Verification items for the finished model (mm, model axes). Face numbers are marked on the shaded views. Give positions to 0.01 mm unless a question says otherwise; leave off trailing zeros. Loops run counter-clockwise (first coordinate to the right, second up) from the corner with the lowest first, then second, coordinate; pieces in that order, holes last. Notation, with made-up numbers: M -7,34.25 L -3,34.25 A6 cw -3,39.25 Z; hole C -21,-4.5 d10. An arc over 180 degrees is marked long. Use a Markdown table: item, result.
from build123d import *

# Parameters (mm, degrees)
SKETCH1_W             = 34.925
SKETCH1_H             = 50.8
BOSS_EXTRUDE1_DEPTH   = 1.5875
F_4_CLEARANCE_HOLE1_D = 3.2639
SKETCH6_W             = 15.875
SKETCH6_H             = 5.588
BOSS_EXTRUDE2_DEPTH   = 1.5875
CUT_EXTRUDE1_DEPTH    = 36.604988506
CUT_EXTRUDE2_DEPTH    = 36.604988506
SKETCH9_W             = 9.573595876
SKETCH9_H             = 10.540114366
CUT_EXTRUDE3_DEPTH    = 36.604988506
FILLET1_R             = 1.016


with BuildPart() as part:
    # Sketch1 → Boss-Extrude1 (new body)
    with BuildSketch(Plane(origin=(0, 0, 0), x_dir=(1, 0, 0), z_dir=(0, 1, 0))):
        Rectangle(SKETCH1_W, SKETCH1_H)
    extrude(amount=BOSS_EXTRUDE1_DEPTH)

    # #4 Clearance Hole1 (through all)
    with Locations(Plane(origin=(0, 1.5875, 0), x_dir=(1, 0, 0), z_dir=(0, 1, 0))):
        with Locations((-14.2875, 22.225), (14.2875, 22.225), (14.2875, -22.225), (-14.2875, -22.225)):
            Hole(F_4_CLEARANCE_HOLE1_D / 2)

    # Sketch6 → Boss-Extrude2 (add)
    with BuildSketch(Plane(origin=(0, 1.5875, 0), x_dir=(1, 0, 0), z_dir=(0, 1, 0))):
        with Locations((0, -28.194)):
            Rectangle(SKETCH6_W, SKETCH6_H)
    extrude(amount=-BOSS_EXTRUDE2_DEPTH)

    # Sketch7 → Cut-Extrude1 (cut, through all)
    with BuildSketch(Plane(origin=(0, 1.5875, 0), x_dir=(1, 0, 0), z_dir=(0, 1, 0))):
        with BuildLine():
            Line((-15.875, 13.8303), (-20.9423, 13.8303))
            Line((-20.9423, 13.8303), (-20.9423, 8.763))
            Line((-20.9423, 8.763), (-20.9423, 3.6957))
            Line((-20.9423, 3.6957), (-15.875, 3.6957))
            ThreePointArc((-15.875, 3.6957), (-10.8077, 8.763), (-15.875, 13.8303))
        make_face()
        with BuildLine():
            Line((12.7, 13.8303), (17.7673, 13.8303))
            Line((17.7673, 13.8303), (17.7673, 8.763))
            Line((17.7673, 8.763), (17.7673, 3.6957))
            Line((17.7673, 3.6957), (12.7, 3.6957))
            ThreePointArc((12.7, 3.6957), (7.6327, 8.763), (12.7, 13.8303))
        make_face()
    extrude(amount=-CUT_EXTRUDE1_DEPTH, mode=Mode.SUBTRACT)

    # Sketch8 → Cut-Extrude2 (cut, through all)
    with BuildSketch(Plane(origin=(0, 1.5875, 0), x_dir=(1, 0, 0), z_dir=(0, 1, 0))):
        with BuildLine():
            Line((6.604, -14.342881029), (6.604, -20.692881029))
            ThreePointArc((6.604, -20.692881029), (5.461, -21.835881029), (4.318, -20.692881029))
            Line((4.318, -20.692881029), (4.318, -14.342881029))
            ThreePointArc((4.318, -14.342881029), (5.461, -13.199881029), (6.604, -14.342881029))
        make_face()
    cut_extrude2 = extrude(amount=-CUT_EXTRUDE2_DEPTH, mode=Mode.SUBTRACT)

    # Mirror1: Cut-Extrude2 across plane
    add(cut_extrude2.mirror(Plane(origin=(0, 0, 0), x_dir=(0, 0, 1), z_dir=(1, 0, 0))), mode=Mode.SUBTRACT)

    # Sketch9 → Cut-Extrude3 (cut, through all)
    with BuildSketch(Plane.XZ):
        with Locations((0, 30.988)):
            Rectangle(SKETCH9_W, SKETCH9_H)
    extrude(amount=-CUT_EXTRUDE3_DEPTH, mode=Mode.SUBTRACT)

    # Fillet1
    fillet1_edges = [part.edges().sort_by_distance(p)[0] for p in [
        (-7.9375, 0.79375, 25.4),
        (7.9375, 0.79375, 25.4),
        (7.9375, 0.79375, 30.988),
        (-7.9375, 0.79375, 30.988),
        (-17.4625, 0.79375, -3.6957),
        (-17.4625, 0.79375, -13.8303),
        (17.4625, 0.79375, -13.8303),
        (17.4625, 0.79375, -3.6957),
        (-17.4625, 0.79375, 25.4),
        (-17.4625, 0.79375, -25.4),
        (17.4625, 0.79375, -25.4),
        (17.4625, 0.79375, 25.4),
    ]]
    fillet(fillet1_edges, radius=FILLET1_R)


solid = part.part
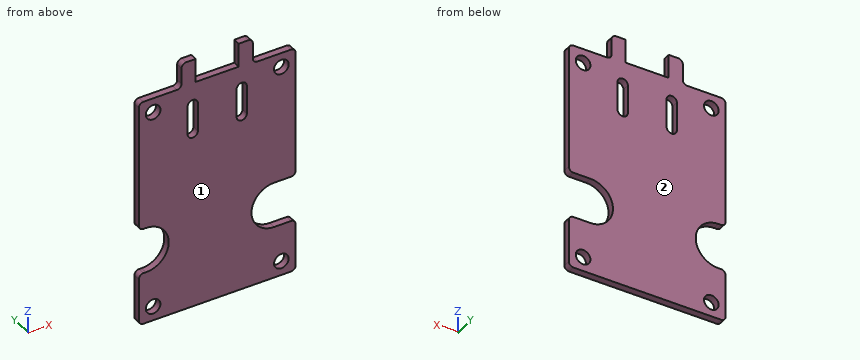
(1) Cross-section at B-B on y = 0.7. State how many separate pieces and enclosed holes the cut face has, then the cut area to 3 significant figures.
Results below:
| item | result |
|---|---|
| separate pieces | 1 |
| enclosed holes | 6 |
| area | 1,590 mm^2 |
(2) Material ranges on line 1 (X direction, y = 0.1, z = 20); line 2 (Z direction, x = -13, y = 1.4); line 3 (Z direction, x = -3.5, y = 1.4), recorded low to high.
Results below:
| item | result |
|---|---|
| line 1 | -17.46 to -6.6, -4.32 to 4.32, 6.6 to 17.46 |
| line 2 | -25.4 to -23.23, -21.22 to -12.94, -4.59 to 21.22, 23.23 to 25.4 |
| line 3 | -25.4 to 25.72 |
(3) Draft check along Y on the marked faces 1 and 2. Enter one of: +Y half, -Y half, draft (parallel to the pull), parting line (faces both ways), or undercut.
Results below:
| item | result |
|---|---|
| face 1 | -Y half |
| face 2 | +Y half |
(4) Gauge pin test, flat ends, axial feed: P1, Ø0.8, axis at y = 1, z = 29, coming from the +X side; P2, Ø0.8, axis at x = 14, y = 0.5, coming from the +Z side; P3, Ø0.5, axis at y = 0.5, z = 28, coming from the -X side; P4, Ø2.5, axis at x = -14.29, z = 22.22, coming from the +Y side. Record the tip position at first contact, or that the pin passes through.
Results below:
| item | result |
|---|---|
| P1 | x = 7.94 |
| P2 | z = 25.4 |
| P3 | x = -7.94 |
| P4 | through |
(5) Cross-section at A-A on z = 19.5. Record the cut outline in (x, y), then the cut area to 3 significant figures.
Results below:
| item | result |
|---|---|
| outline | M -17.46,0 L -6.6,0 L -6.6,1.59 L -17.46,1.59 Z; M -4.32,0 L 4.32,0 L 4.32,1.59 L -4.32,1.59 Z; M 6.6,0 L 17.46,0 L 17.46,1.59 L 6.6,1.59 Z |
| area | 48.2 mm^2 |
